The listing builds one solid part. Answer for the finished solid, in the listing's coordinates (mm). A direction names the side the tool comes from. Coordinates: 2 decimals unless noted, no trailing zeros. Order: outer loops, then holes, each group sorted by start corner. A loop starts at its lowest first (then second) coordinate and runs counter-clockwise, first axis right, second up. Notation, with made-up numbers: (25.25, 28) -> (45.25, 28) arc R25 ccw to (45.25, 62) -> close; hole circle Ø10 at (43, -2). An arc over 180 degrees is marked (long way). Return JSON: item names as keys, results as strings.
Autodesk Inventor part; units mm, degrees
ref_plane "YZ Plane" through (0, 0, 0) normal (1, 0, 0) x (0, 1, 0)
ref_plane "XZ Plane" through (0, 0, 0) normal (0, 1, 0) x (-1, 0, 0)
ref_plane "XY Plane" through (0, 0, 0) normal (0, 0, 1) x (1, 0, 0)
sketch "スケッチ1" plane through (0, 0, 0) normal (0, 0, 1) x (1, 0, 0)
  circle A0 centre (0, 0) radius 35
  circle A1 centre (0, 0) radius 33
  line L0 (-45, 40) -> (45, 40)
  line L1 (45, 40) -> (45, -40)
  line L2 (45, -40) -> (-45, -40)
  line L3 (-45, -40) -> (-45, 40)
  line L4 (-45, 40) -> (45, -40) construction
  line L5 (45, 40) -> (-45, -40) construction
  dimension "d0" = 70
  dimension "d1" = 66
  dimension "d2" = 90
  dimension "d3" = 80
extrude "押し出し1" add sketch "スケッチ1" along normal blind 3 contours L0 L1 L2 L3
sketch "スケッチ2" plane through (0, 0, 3) normal (0, 0, 1) x (1, 0, 0)
  circle A0 centre (0, 0) radius 35
  circle A1 centre (0, 0) radius 35
  circle A2 centre (0, 0) radius 33
  dimension "d6" = 66
extrude "押し出し2" add sketch "スケッチ2" along normal blind 3 and the other way blind 3
sketch "スケッチ3" plane through (0, 0, 6) normal (0, 0, 1) x (1, 0, 0)
  circle A0 centre (0, 0) radius 33
  circle A1 centre (0, 0) radius 35
extrude "押し出し3" add sketch "スケッチ3" along normal blind 59
sketch "スケッチ4" plane through (0, 0, 65) normal (0, 0, 1) x (1, 0, 0)
  circle A0 centre (0, 0) radius 33
  circle A1 centre (0, 0) radius 35
sketch "スケッチ5" plane through (0, 0, 0) normal (0, 0, -1) x (-1, 0, 0)
  line L0 (-45, 40) -> (-35, 40)
  line L1 (-35, 40) -> (-35, 30)
  line L2 (-35, 30) -> (-45, 30)
  line L3 (-45, 30) -> (-45, 40)
  line L4 (-45, -40) -> (-35, -40)
  line L5 (-35, -40) -> (-35, -30)
  line L6 (-35, -30) -> (-45, -30)
  line L7 (-45, -30) -> (-45, -40)
  line L8 (45, -40) -> (35, -40)
  line L9 (35, -40) -> (35, -30)
  line L10 (35, -30) -> (45, -30)
  line L11 (45, -30) -> (45, -40)
  line L12 (45, 40) -> (35, 40)
  line L13 (35, 40) -> (35, 30)
  line L14 (35, 30) -> (45, 30)
  line L15 (45, 30) -> (45, 40)
  dimension "d13" = 10
  dimension "d14" = 10
  dimension "d15" = 10
  dimension "d16" = 10
  dimension "d17" = 10
  dimension "d18" = 10
  dimension "d19" = 10
hole "穴1" at (35, 30, 0) at (-35, 30, 0) at (-35, -30, 0) at (35, -30, 0) direction (0, 0, 1) diameter 3 depth 8 tip angle 118
properties part number "知能ロボコン発射口ver2"
Item 1: Determine the mould class of faces 3 (the flat face through (-31, 18, 3)), 4 (the flat face through (-45, -1, 1)), 5 (the cylindrical face through (35.9, -31.2, 1.5)) for opening direction X: pulls with the +X half, pulls with the -X half, needs draft (parallel to the pull), parting line crosses it, or undercut.
Answer list:
{"face 3": "needs draft", "face 4": "pulls with the -X half", "face 5": "undercut"}
Item 2: The part is cut by section C-C on y = 30. Determine the outline of the cut face in (x, z), plus the area to 3 significant figures.
Answer list:
{"outline": "(-45, 0) -> (-36.5, 0) -> (-36.5, 3) -> (-45, 3) -> close; (-33.5, 0) -> (-13.75, 0) -> (-13.75, 65) -> (-18.03, 65) -> (-18.03, 3) -> (-33.5, 3) -> close; (13.75, 0) -> (33.5, 0) -> (33.5, 3) -> (18.03, 3) -> (18.03, 65) -> (13.75, 65) -> close; (36.5, 0) -> (45, 0) -> (45, 3) -> (36.5, 3) -> close", "area": "700 mm2"}
Item 3: The part is cut by section D-D on z = 29. Determine the outline of the cut face in (x, y), plus the area to 3 significant figures.
Answer list:
{"outline": "circle Ø70 at (0, 0); hole circle Ø66 at (0, 0)", "area": "427 mm2"}
Item 4: The part is cut by section A-A on x = 6.5. Determine the outline of the cut face in (y, z), plus the area to 3 significant figures.
Answer list:
{"outline": "(-40, 0) -> (-32.35, 0) -> (-32.35, 65) -> (-34.39, 65) -> (-34.39, 3) -> (-40, 3) -> close; (32.35, 0) -> (40, 0) -> (40, 3) -> (34.39, 3) -> (34.39, 65) -> (32.35, 65) -> close", "area": "299 mm2"}
Item 5: Flat-ended cylindrical pins translate along their axes: pin 1 (4 mm diameter, centred on y = 10.5, z = 11.5, fed in from -X); pin 2 (3.5 mm diameter, centred on x = 35, y = 30, fed in from -Z); pin 3 (10 mm diameter, centred on x = -7.5, z = 50, fed in from -Y); pin 4 (5 mm diameter, centred on x = -35, y = 30, fed in from +Z). Find the tip coordinate at first contact, or state that the pin passes through.
Answer list:
{"pin 1": "x = -33.95", "pin 2": "z = 0", "pin 3": "y = -34.91", "pin 4": "z = 3"}
Item 6: Which of the six approach directions +Z, -Z, +X, -X, +Y, -Y give full straight-line access (tool end or side, diameter ignored) to faces 1 (the flat face through (-1, 40, 1)), 2 (the cylindrical face through (-28, 21, 34))?
Answer list:
{"face 1": "+Z, -Z, +X, -X, +Y", "face 2": "+Z"}
Item 7: Find the intervals of material crossed by probe 1 along Y at (x, z) = (35, 1.2); probe 2 along X at (y, z) = (30, 2); probe 3 along Y at (x, z) = (0, 27), in increasing order.
Answer list:
{"probe 1": "-40 to -31.5, -28.5 to 28.5, 31.5 to 40", "probe 2": "-45 to -36.5, -33.5 to -13.75, 13.75 to 33.5, 36.5 to 45", "probe 3": "-35 to -33, 33 to 35"}
Item 8: The part is cut by section B-B on y = -17. Determine the outline of the cut face in (x, z).
Answer list:
{"outline": "(-45, 0) -> (-28.28, 0) -> (-28.28, 65) -> (-30.59, 65) -> (-30.59, 3) -> (-45, 3) -> close; (28.28, 0) -> (45, 0) -> (45, 3) -> (30.59, 3) -> (30.59, 65) -> (28.28, 65) -> close"}
